Can you work these out from the model? Positions are in its coordinate system, mm. Coordinates: 2 decimals unless noted, no trailing zeros. Write each loop counter-clockwise with the first axis right and the second up, starting at its lowest first coordinate (ties: lowest second). Pieces come first, ordered by that corner, then holes.
Solid Edge part; units mm, degrees
sketch "Sketch1" plane through (0, 0, 0) normal (0, 0, 1) x (1, 0, 0)
  circle A0 centre (0, 0) radius 7.5
extrude "ExtrudedProtrusion_1" add sketch "Sketch1" along normal blind 300 and the other way blind 55
sketch "Sketch2" plane through (0, 0, 0) normal (0, 0, 1) x (1, 0, 0)
  line L0 (-1.5, 6.5) -> (1.5, 6.5)
  line L1 (1.5, 6.5) -> (1.5, 8.5)
  line L2 (1.5, 8.5) -> (-1.5, 8.5)
  line L3 (-1.5, 8.5) -> (-1.5, 6.5)
  dimension "D1" = 1.5
extrude "ExtrudedProtrusion_2" add sketch "Sketch2" along normal blind 30
sketch "Sketch3" plane through (0, 0, 300) normal (0, 0, 1) x (0, 1, 0)
  line L0 (1.5023, 6.5) -> (-1.5023, 6.5)
  line L1 (-1.5023, 6.5) -> (-1.5023, 8.5)
  line L2 (-1.5023, 8.5) -> (1.5023, 8.5)
  line L3 (1.5023, 8.5) -> (1.5023, 6.5)
  dimension "D1" = 1.5023
  dimension "D2" = 1.5023
extrude "ExtrudedProtrusion_3" add sketch "Sketch3" against normal blind 30
1. If I drill on L1, parallel to Y at x = -1.5, z = 113.5; L2, parallel to Y at x = 1, z = 33.5; L3, parallel to X at y = -3.25, z = 120.5, over which ranges is the centre line in solid material (lowest first)?
2. If we section it at B-B, the plane y = -5: List the corners of the cut face in (x, z) for me, plus the area to 3 significant figures.
3. We'd pull the mould along Y, two halves only. Please class faces 1 (the face through (7.154, -2.253, 120.015)), 2 (the face through (0, 0, -55)): released by +Y, released by -Y, zero draft, split by the parting line, or undercut.
4. If we section it at A-A, the plane z = 110: List the corners of the cut face in (x, y) for me.
5. I'm going to push flat-ended pins straight in: P1, Ø1, axis at y = 6.5, z = 79.5, coming from the +X side; P2, Ø4, axis at x = 5, z = -14, coming from the +Y side; P3, Ø0.9, axis at y = 8, z = 12, coming from the -X side. Where does each tip first touch, or does it pass through?
Answers:
1. L1: y = -7.35 to 7.35
1. L2: y = -7.43 to 7.43
1. L3: x = -6.76 to 6.76
2. outline: (-5.59, -55) - (5.59, -55) - (5.59, 300) - (-5.59, 300) - close
2. area: 3,970 mm2
3. face 1: split by the parting line
3. face 2: zero draft
4. outline: circle Ø15 at (0, 0)
5. P1: stops at x = 4.5
5. P2: stops at y = 6.87
5. P3: stops at x = -1.5
